Input: part model. Units: mm. Frame: model coordinates. Give positions to 0.01 mm unless a question says otherwise; leave off trailing zeros. Loops run counter-clockwise (first coordinate to the right, second up) from the corner with the lowest first, then second, coordinate; pieces in that order, holes last. Notation, with made-up numbers: (83.5, 52.25) - (90.5, 52.25) arc R18 ccw to (90.5, 63.25) - close; hole circle Ø2 at (24.25, 88.5). An arc over 180 degrees is marked (long way). Answer as a JSON object with one key per item and string values.
from build123d import *

# Parameters (mm, degrees)
SKETCH_1_W          = 50
SKETCH_1_H          = 30
EXTRUDE_1_DEPTH     = 6.5
CUT_EXTRUDE_1_DEPTH = 30.870554062
SKETCH_4_R          = 1.55
CUT_EXTRUDE_2_DEPTH = 30.870554062
SKETCH_5_R          = 1.5
CUT_EXTRUDE_3_DEPTH = 40.588508434


with BuildPart() as part:
    # 草图1 → 凸台-拉伸1 (new body)
    with BuildSketch(Plane.XY):
        Rectangle(SKETCH_1_W, SKETCH_1_H)
    extrude(amount=EXTRUDE_1_DEPTH)

    # 草图2 → 切除-拉伸1 (cut, through all)
    with BuildSketch(Plane.XY.offset(6.5)):
        with BuildLine():
            ThreePointArc((-3.55, 4.95), (-5.939949494, 5.939949494), (-4.95, 3.55))
            Line((-4.95, 3.55), (-4.95, 4.95))
            Line((-4.95, 4.95), (-3.55, 4.95))
        make_face()
        with BuildLine():
            Line((-4.95, 4.95), (-4.95, 3.55))
            ThreePointArc((-4.95, 3.55), (-3.960050506, 3.960050506), (-3.55, 4.95))
            Line((-3.55, 4.95), (-4.95, 4.95))
        make_face()
        with BuildLine():
            ThreePointArc((3.55, 4.95), (3.960050506, 3.960050506), (4.95, 3.55))
            Line((4.95, 3.55), (4.95, 4.95))
            Line((4.95, 4.95), (3.55, 4.95))
        make_face()
        with BuildLine():
            Line((4.95, 4.95), (4.95, 3.55))
            ThreePointArc((4.95, 3.55), (5.939949494, 3.960050506), (6.35, 4.95))
            ThreePointArc((6.35, 4.95), (4.95, 6.35), (3.55, 4.95))
            Line((3.55, 4.95), (4.95, 4.95))
        make_face()
        with BuildLine():
            ThreePointArc((4.95, -3.55), (3.960050506, -3.960050506), (3.55, -4.95))
            Line((3.55, -4.95), (4.95, -4.95))
            Line((4.95, -4.95), (4.95, -3.55))
        make_face()
        with BuildLine():
            Line((4.95, -4.95), (3.55, -4.95))
            ThreePointArc((3.55, -4.95), (4.95, -6.35), (6.35, -4.95))
            ThreePointArc((6.35, -4.95), (5.939949494, -3.960050506), (4.95, -3.55))
            Line((4.95, -3.55), (4.95, -4.95))
        make_face()
        with BuildLine():
            ThreePointArc((-4.95, -3.55), (-5.939949494, -5.939949494), (-3.55, -4.95))
            Line((-3.55, -4.95), (-4.95, -4.95))
            Line((-4.95, -4.95), (-4.95, -3.55))
        make_face()
        with BuildLine():
            Line((-4.95, -4.95), (-3.55, -4.95))
            ThreePointArc((-3.55, -4.95), (-3.960050506, -3.960050506), (-4.95, -3.55))
            Line((-4.95, -3.55), (-4.95, -4.95))
        make_face()
    extrude(amount=-CUT_EXTRUDE_1_DEPTH, mode=Mode.SUBTRACT)

    # 草图4 → 切除-拉伸2 (cut, through all)
    with BuildSketch(Plane(origin=(0, 0, 0), x_dir=(-1, 0, 0), z_dir=(0, 0, -1))):
        with Locations((-17, 10)):
            Circle(SKETCH_4_R)
        with Locations((-17, -10)):
            Circle(SKETCH_4_R)
        with Locations((17, -10)):
            Circle(SKETCH_4_R)
        with Locations((17, 10)):
            Circle(SKETCH_4_R)
    extrude(amount=-CUT_EXTRUDE_2_DEPTH, mode=Mode.SUBTRACT)

    # 草图5 → 切除-拉伸3 (cut, through all)
    with BuildSketch(Plane(origin=(0, 15, 0), x_dir=(1, 0, 0), z_dir=(0, 1, 0))):
        with Locations(Location((-10, -4, 0), (0, 0, 180))):
            Circle(SKETCH_5_R)
        with Locations(Location((0, -4, 0), (0, 0, 180))):
            Circle(SKETCH_5_R)
        with Locations(Location((10, -4, 0), (0, 0, 180))):
            Circle(SKETCH_5_R)
    extrude(amount=-CUT_EXTRUDE_3_DEPTH, mode=Mode.SUBTRACT)


solid = part.part
Item 1: Cut plane D-D (z = 3). Give the number of separate pieces and of enclosed holes in the cut face, then the cut area to 3 significant figures.
Geometry check:
{"separate pieces": "4", "enclosed holes": "8", "area": "1,240 mm2"}
Item 2: Cut plane A-A (x = -10). Return loops of the section in (y, z), then the cut area to 3 significant figures.
Geometry check:
{"outline": "(-15, 0) - (15, 0) - (15, 2.5) - (-15, 2.5) - close; (-15, 5.5) - (15, 5.5) - (15, 6.5) - (-15, 6.5) - close", "area": "105 mm2"}
Item 3: Cut plane B-B (y = -10). Return loops of the section in (x, z).
Geometry check:
{"outline": "(-25, 0) - (-18.55, 0) - (-18.55, 6.5) - (-25, 6.5) - close; (-15.45, 0) - (15.45, 0) - (15.45, 6.5) - (-15.45, 6.5) - close; (18.55, 0) - (25, 0) - (25, 6.5) - (18.55, 6.5) - close; hole circle Ø3 at (-10, 4); hole circle Ø3 at (0, 4); hole circle Ø3 at (10, 4)"}
Item 4: Mould query, pull axis X, two halves, no side actions, for faces 1 (the face through (-25, 0, 3)), 2 (the face through (0, 0, 6.5)), 3 (the face through (-1.43, 0.21, 4.45)). Classes: released by +X, released by -X, zero draft, split by the parting line, or undercut.
Geometry check:
{"face 1": "released by -X", "face 2": "zero draft", "face 3": "undercut"}
Item 5: Contact query for a flat-ended pin moving along its axis: P1, Ø2, axis at x = 8.5, y = 0, coming from the -Z side. Output: stop coordinate, or through.
Geometry check:
{"P1": "stops at z = 0"}
Item 6: Cut plane C-C (x = 17). Return loops of the section in (y, z), then the cut area to 3 significant figures.
Geometry check:
{"outline": "(-15, 0) - (-11.55, 0) - (-11.55, 6.5) - (-15, 6.5) - close; (-8.45, 0) - (8.45, 0) - (8.45, 6.5) - (-8.45, 6.5) - close; (11.55, 0) - (15, 0) - (15, 6.5) - (11.55, 6.5) - close", "area": "155 mm2"}
Item 7: Material intervals for line 1 (Y direction, x = -17, z = 2.75); line 2 (X direction, y = 4.95, z = 2); line 3 (Y direction, x = -4.95, z = 3.25), sorted ascending. Write a range as [from, to].
Geometry check:
{"line 1": "y = [-15, -11.55], [-8.45, 8.45], [11.55, 15]", "line 2": "x = [-25, -6.35], [-3.55, 3.55], [6.35, 25]", "line 3": "y = [-15, -6.35], [-3.55, 3.55], [6.35, 15]"}
